Build history of the part. All positions in model axes, mm. Face numbers are marked on the shaded views. Give positions to 0.01 mm unless a question says otherwise; leave off trailing zeros. Order: outer loops, then holes, each group sorted by start corner. A loop starts at its lowest first (then second) coordinate and runs counter-clockwise, first axis right, second up. Notation, with made-up numbers: (-5, 53.5) -> (51, 53.5) arc R27 cw to (51, 77.5) -> close; hole circle Ø5 at (72, -17.75). An arc over 180 degrees is marked (long way). One line per question, with ' | ' between items. Start each with the question number.
(1) Cut at A-A (z = -30). Give the cut face in (x, y).
(2) Cut at C-C (z = 15). Give the cut face in (x, y), then the cut area to 3 significant figures.
(3) Drill centre lines: L1, parallel to X at y = 7.25, z = 15; L2, parallel to X at y = 3.75, z = 19; L3, parallel to X at y = 6.75, z = -30. Where is each one in solid material? Low to high. Write a range as from..to.
(4) Cut at B-B (x = 0). Give the cut face in (y, z), then the cut area to 3 significant figures.
(5) Pull direction X, two halves, no side cores. Call the marked faces 1, 2 and 3: +X half, -X half, draft (parallel to the pull), parting line (faces both ways), or undercut.
(6) Cut at D-D (y = 8.25). Give the cut face in (x, z), then the cut area to 3 significant figures.
(7) Pin check, flat tips, straight feed: pin 1 Ø3 at (x, y) = (-24, 8) entering from +Z; pin 2 Ø6 at (x, z) = (0, -30) entering from +Y; pin 3 Ø1.5 at (y, z) = (1.5, -12) entering from +X; pin 4 Ø4 at (x, y) = (-9.5, 1) entering from -Z. Stop position of each tip, or through.
from build123d import *

# Parameters (mm, degrees)
SKETCH1_R           = 10
SKETCH1_R_2         = 5
BOSS_EXTRUDE1_DEPTH = 10


with BuildPart() as part:
    # Sketch1 → Boss-Extrude1 (new body)
    with BuildSketch(Plane(origin=(0, 0, 0), x_dir=(1, 0, 0), z_dir=(0, 1, 0))):
        with BuildLine():
            ThreePointArc((-9.400507195, 26.58965332), (-11.173070065, 6.45077501), (-27.72756885, -5.153748621))
            ThreePointArc((-27.72756885, -5.153748621), (-34.641016151, -20), (-18.327061655, -21.435904699))
            ThreePointArc((-18.327061655, -21.435904699), (0, -12.901550019), (18.327061655, -21.435904699))
            ThreePointArc((18.327061655, -21.435904699), (34.641016151, -20), (27.72756885, -5.153748621))
            ThreePointArc((27.72756885, -5.153748621), (11.173070065, 6.45077501), (9.400507195, 26.58965332))
            ThreePointArc((9.400507195, 26.58965332), (0, 40), (-9.400507195, 26.58965332))
        make_face()
        with Locations(Location((0, 0, 0), (0, 0, 270))):
            Circle(SKETCH1_R, mode=Mode.SUBTRACT)
        with Locations(Location((25.980762114, -15, 0), (0, 0, 270))):
            Circle(SKETCH1_R_2, mode=Mode.SUBTRACT)
        with Locations(Location((0, 30, 0), (0, 0, 270))):
            Circle(SKETCH1_R_2, mode=Mode.SUBTRACT)
        with Locations(Location((-25.980762114, -15, 0), (0, 0, 270))):
            Circle(SKETCH1_R_2, mode=Mode.SUBTRACT)
    extrude(amount=BOSS_EXTRUDE1_DEPTH)


solid = part.part
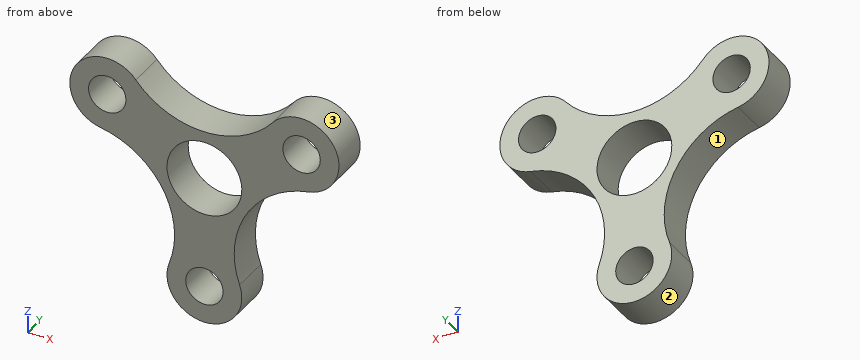
Result set:
1) outline: (-10, 0) -> (-5, 0) -> (-5, 10) -> (-10, 10) -> close; (5, 0) -> (10, 0) -> (10, 10) -> (5, 10) -> close
2) outline: (-35.98, 0) -> (-30.98, 0) -> (-30.98, 10) -> (-35.98, 10) -> close; (-20.98, 0) -> (-9.8, 0) -> (-9.8, 10) -> (-20.98, 10) -> close; (9.8, 0) -> (20.98, 0) -> (20.98, 10) -> (9.8, 10) -> close; (30.98, 0) -> (35.98, 0) -> (35.98, 10) -> (30.98, 10) -> close | area: 324 mm2
3) L1: x = -35.98..-30.98, -20.98..-9.8, 9.8..20.98, 30.98..35.98 | L2: x = -35.15..-28.98, -22.98..-15.96, 15.96..22.98, 28.98..35.15 | L3: x = -10..-5, 5..10
4) outline: (0, -40) -> (10, -40) -> (10, -35) -> (0, -35) -> close; (0, -25) -> (10, -25) -> (10, -10) -> (0, -10) -> close; (0, 10) -> (10, 10) -> (10, 12.9) -> (0, 12.9) -> close | area: 229 mm2
5) face 1: -X half | face 2: parting line | face 3: undercut
6) outline: (-27.73, 5.15) arc R23.95 cw to (-9.4, -26.59) arc R10 ccw (long way) to (9.4, -26.59) arc R23.95 cw to (27.73, 5.15) arc R10 ccw (long way) to (18.33, 21.44) arc R23.95 cw to (-18.33, 21.44) arc R10 ccw (long way) to start; hole circle Ø10 at (-25.98, 15); hole circle Ø20 at (0, 0); hole circle Ø10 at (0, -30); hole circle Ø10 at (25.98, 15) | area: 1,400 mm2
7) pin 1: stops at z = 24.99 | pin 2: passes through | pin 3: stops at x = 9.06 | pin 4: stops at z = -36.61
